Read the model definition and answer for the solid it produces. Units are mm, in the model's axes. Give positions to 0.01 mm unless a question says otherwise; leave off trailing zeros. Write each loop counter-clockwise with the first axis right and the second up, starting at its lowest first coordinate (ties: lowest second). Pieces come first, ordered by that corner, then holes.
```python
from build123d import *

# Parameters (mm, degrees)
BOSS_EXTRUDE1_DEPTH = 2.54


with BuildPart() as part:
    # Sketch1 → Boss-Extrude1 (new body, symmetric)
    with BuildSketch(Plane(origin=(0, 0, 0), x_dir=(1, 0, 0), z_dir=(0, 1, 0))):
        Polygon((12.7, 152.4), (-12.7, 152.4), (-12.7, 147.32), (-38.1, 147.32), (-38.1, 152.4), (-63.5, 152.4), (-63.5, 147.32), (-88.9, 147.32), (-88.9, 152.4), (-114.3, 152.4), (-114.3, 147.32), (-139.7, 147.32), (-139.7, 152.4), (-152.4, 152.4), (-152.4, 139.7), (-147.32, 139.7), (-147.32, 114.3), (-152.4, 114.3), (-152.4, 88.9), (-147.32, 88.9), (-147.32, 63.5), (-152.4, 63.5), (-152.4, 38.1), (-147.32, 38.1), (-147.32, 12.7), (-152.4, 12.7), (-152.4, -12.7), (-147.32, -12.7), (-147.32, -38.1), (-152.4, -38.1), (-152.4, -63.5), (-147.32, -63.5), (-147.32, -88.9), (-152.4, -88.9), (-152.4, -114.3), (-147.32, -114.3), (-147.32, -139.7), (-152.4, -139.7), (-152.4, -152.4), (-139.7, -152.4), (-139.7, -147.32), (-114.3, -147.32), (-114.3, -152.4), (-88.9, -152.4), (-88.9, -147.32), (-63.5, -147.32), (-63.5, -152.4), (-38.1, -152.4), (-38.1, -147.32), (-12.7, -147.32), (-12.7, -152.4), (12.7, -152.4), (12.7, -147.32), (38.1, -147.32), (38.1, -152.4), (63.5, -152.4), (63.5, -147.32), (88.9, -147.32), (88.9, -152.4), (114.3, -152.4), (114.3, -147.32), (139.7, -147.32), (139.7, -152.4), (152.4, -152.4), (152.4, -139.7), (147.32, -139.7), (147.32, -114.3), (152.4, -114.3), (152.4, -88.9), (147.32, -88.9), (147.32, -63.5), (152.4, -63.5), (152.4, -38.1), (147.32, -38.1), (147.32, -12.7), (152.4, -12.7), (152.4, 12.7), (147.32, 12.7), (147.32, 38.1), (152.4, 38.1), (152.4, 63.5), (147.32, 63.5), (147.32, 88.9), (152.4, 88.9), (152.4, 114.3), (147.32, 114.3), (147.32, 139.7), (152.4, 139.7), (152.4, 152.4), (139.7, 152.4), (139.7, 147.32), (114.3, 147.32), (114.3, 152.4), (88.9, 152.4), (88.9, 147.32), (63.5, 147.32), (63.5, 152.4), (38.1, 152.4), (38.1, 147.32), (12.7, 147.32), align=None)
    extrude(amount=BOSS_EXTRUDE1_DEPTH, both=True)


solid = part.part
```
Item 1: Each of these flat-tipped pins is pushed along its axis until it touches: pin 1 Ø1.5 at (y, z) = (-0.5, 29.5) entering from -X; pin 2 Ø1 at (x, y) = (119.5, 0.5) entering from -Z. Where does it stop, or does it pass through?
Result set:
pin 1: stops at x = -147.32
pin 2: stops at z = -147.32
Item 2: Section B-B (z = 81.5) is taken. Write down the section's boundary in (x, y), and give its area (3 significant figures).
Result set:
outline: (-147.32, -2.54) - (147.32, -2.54) - (147.32, 2.54) - (-147.32, 2.54) - close
area: 1,500 mm2
Item 3: Section A-A (x = -68.5) is taken. Write down the section's boundary in (y, z), and give its area (3 significant figures).
Result set:
outline: (-2.54, -147.32) - (2.54, -147.32) - (2.54, 147.32) - (-2.54, 147.32) - close
area: 1,500 mm2
Item 4: Find the intervals of material crossed by line 1 along X through (y, z) = (1.9, -138), in increasing order.
Result set:
line 1: x = -147.32 to 147.32
